Design review of the part built by this model. Coordinates are the model's own, in mm. A direction names the side the tool comes from. Coordinates: 2 decimals unless noted, no trailing zeros. Loops run counter-clockwise (first coordinate to the right, second up) from the corner with the lowest first, then second, coordinate; pieces in that order, holes last. Notation, with made-up numbers: (50.25, 27) -> (58.25, 27) arc R29 cw to (58.25, 66) -> close; hole circle Ø3 at (-21.5, 46.5). An arc over 180 degrees is marked (long way). Use a Markdown table: item, result. Add a question column.
Q1. Draft analysis for pull direction Z (two halves, no side actions). For faces 1 (the face through (20, 85, -8.765)), 2 (the face through (29.93, 37.543, 74.263)), 3 (the face through (25, 80, -2)), state which applies: pulls with the +Z half, pulls with the -Z half, needs draft (parallel to the pull), parting line crosses it, or undercut.
Q2. Take a section at C-C on y = -85. Write out the cut boundary in (x, z), plus the area to 3 significant figures.
Q3. Take a section at A-A on y = 0. Write out the cut boundary in (x, z).
Q4. For probe 1 along Y at (x, z) = (14.5, -0.5); probe 2 along X at (y, z) = (-86.5, 31), list the stretches that pass through material, from the lowest coordinate up.
Q5. Take a section at D-D on x = 22.5. Count the separate pieces of the cut face and the enclosed holes in it, plus the area to 3 significant figures.
Q6. For faces 4 (the face through (19.93, -49.964, -77.898)), 5 (the face through (19.93, 35.036, 69.326)), 6 (the face through (19.93, 49.964, -77.898)), 7 (the face through (19.93, -92.444, 4.321)), list the 3-axis set-ups (+Z, -Z, +X, -X, +Y, -Y) from which the entire face can be reached by the end or side of a thin tool; tool diameter is ignored.
Q7. Take a section at B-B on z = 13.5. Write out the cut boundary in (x, y).
Q8. Clearance check with flat-ended pins moving along their axes: pin 1 Ø1.5 at (x, z) = (13, -84.5) entering from -Y; pin 2 Ø10.5 at (x, y) = (17.5, 83) entering from -Z; pin 3 Ø10.5 at (x, y) = (19, 84.5) entering from +Z. State where each tip first meets the part, or that it passes through.
Autodesk Inventor part; units mm, degrees
ref_plane "YZ Plane" through (0, 0, 0) normal (1, 0, 0) x (0, 1, 0)
ref_plane "XZ Plane" through (0, 0, 0) normal (0, 1, 0) x (-1, 0, 0)
ref_plane "XY Plane" through (0, 0, 0) normal (0, 0, 1) x (1, 0, 0)
sketch "Skizze1" plane through (0, 0, 0) normal (1, 0, 0) x (0, 1, 0)
  circle A0 centre (0, 0) radius 40
  circle A1 centre (0, 0) radius 108
  dimension "d0" = 216
  dimension "d1" = 80
extrude "Extrusion1" add sketch "Skizze1" along normal blind 15
sketch "Skizze3" plane through (15, 0, 0) normal (1, 0, 0) x (0, 0, -1)
  circle A0 centre (0, -85) radius 10 construction
  line L0 (0, -95) -> (-8.7647, -89.8146)
  line L1 (-8.7647, -80.1854) -> (0, -75)
  line L2 (0, -75) -> (8.7647, -80.1854)
  line L3 (8.7647, -80.1854) -> (8.7647, -89.8146)
  line L4 (0, -95) -> (8.7647, -89.8146)
  line L5 (-8.7647, -80.1854) -> (-8.7647, -89.8146)
  point P0 (0, 0)
  dimension "d8" = 20
  dimension "d9" = 85
extrude "Extrusion3" add sketch "Skizze3" along normal blind 10
sketch "Skizze4" plane through (25, 0, 0) normal (1, 0, 0) x (0, 0, -1)
  circle A0 centre (0, -85) radius 5
  point P0 (0, 0)
  dimension "d12" = 10
extrude "Extrusion4" add sketch "Skizze4" along normal blind 10
pattern_circular "Runde Anordnung1" count 6 over 360 about axis through (-10, 0, 0) along (1, 0, 0) of "Extrusion3", "Extrusion4"
properties part number "DN80-Flansch"
Answer list:
| question | item | result |
|---|---|---|
| 1 | face 1 | pulls with the -Z half |
| 1 | face 2 | undercut |
| 1 | face 3 | needs draft |
| 2 | outline | (0, -66.63) -> (15, -66.63) -> (15, -8.76) -> (25, -8.76) -> (25, -5) -> (35, -5) -> (35, 5) -> (25, 5) -> (25, 8.76) -> (15, 8.76) -> (15, 66.63) -> (0, 66.63) -> close |
| 2 | area | 2,270 mm² |
| 3 | outline | (0, -108) -> (15, -108) -> (15, -40) -> (0, -40) -> close; (0, 40) -> (15, 40) -> (15, 108) -> (0, 108) -> close |
| 4 | probe 1 | -108 to -40, 40 to 108 |
| 4 | probe 2 | 0 to 15 |
| 5 | separate pieces | 6 |
| 5 | enclosed holes | 0 |
| 5 | area | 1,560 mm² |
| 6 | face 4 | -Z, +X, -Y |
| 6 | face 5 | +X |
| 6 | face 6 | -Z, +X, +Y |
| 6 | face 7 | +Z, +X, -Y |
| 7 | outline | (0, -107.15) -> (15, -107.15) -> (15, -37.65) -> (0, -37.65) -> close; (0, 37.65) -> (15, 37.65) -> (15, 107.15) -> (0, 107.15) -> close |
| 8 | pin 1 | y = -68.19 |
| 8 | pin 2 | z = -74.3 |
| 8 | pin 3 | z = 71.32 |
